from build123d import *

# Parameters (mm, degrees)
F0_W     = 32
F0_H     = 50
F0_W_2   = 2
F0_H_2   = 6
F1_DEPTH = 10
F2_R     = 0.5


with BuildPart() as f1:
    # F0 (on Top) → F1 (new body)
    with BuildSketch(Plane.XY):
        Polygon((-17.5, 26.5), (-17.5, 25), (-17.5, -26.5), (17.5, -26.5), (17.5, 26.5), (-16, 26.5), align=None)
        Rectangle(F0_W, F0_H, mode=Mode.SUBTRACT)
        Polygon((-38, 25), (-17.5, 25), (-17.5, 26.5), (-39.5, 26.5), (-39.5, -8.5), (-38, -8.5), (-38, -2.5), align=None)
        with Locations((-37, -5.5)):
            Rectangle(F0_W_2, F0_H_2)
    extrude(amount=F1_DEPTH)

    # F2
    f2_edges = [f1.edges().sort_by_distance(p)[0] for p in [
        (-36, -2.5, 5),
        (-36, -8.5, 5),
        (17.5, -26.5, 5),
        (17.5, 26.5, 5),
        (-17.5, -26.5, 5),
        (-39.5, 26.5, 5),
        (-39.5, -8.5, 5),
    ]]
    fillet(f2_edges, radius=F2_R)


solid = f1.part
Work out the finished part from the listing and answer in its coordinate system (mm). A direction names the side the tool comes from. Round coordinates to 2 decimals unless told otherwise and drop trailing zeros. Write each loop counter-clockwise with the first axis right and the second up, starting at its lowest first coordinate (ties: lowest second). Pieces come first, ordered by that corner, then holes. Notation, with made-up numbers: (11, -15) -> (41, -15) arc R23 cw to (41, 17) -> close; hole circle Ø11 at (43.5, 52.25). An arc over 180 degrees is marked (long way). Answer as CSV lines item,"result". Start each with the question number.
(1) The part is cut by section A-A, the plane y = -13.5. Give the vertices of the cut face in (x, z).
(2) This flat-tipped pin is pushed along its axis until it touches: pin 1 (3 mm diameter, centred on x = -37, z = 6.5, fed in from -Y). Where does it stop, or does it pass through?
(3) The part is cut by section D-D, the plane y = 13.5. Give the vertices of the cut face in (x, z).
(4) The part is cut by section B-B, the plane x = -2. Give the vertices of the cut face in (y, z).
(5) The part is cut by section C-C, the plane z = 8. Give the vertices of the cut face in (x, y), then the cut area to 3 significant figures.
(6) A tool of negligible diameter and unlimited length cuts with its end or side. For faces 4 (the flat face through (-17.5, 0, 5)), 5 (the flat face through (-17, 4, 10)), 6 (the flat face through (-37, -2.5, 5)), 7 (the flat face through (-38, -8.5, 5)), from which of +Z, -Z, +X, -X, +Y, -Y can it reach the whole face along a straight path? Write none if from no direction.
(7) The mould has two halves that part along X. Classify faces 1 (the flat face through (-39.5, 9, 5)), 2 (the flat face through (-17, 4, 0)), 3 (the flat face through (-16, 0, 5)): +X half, -X half, draft (parallel to the pull), parting line (faces both ways), or undercut.
(8) Find the intervals of material crossed by probe 1 along X at (y, z) = (15.5, 4.5); probe 2 along X at (y, z) = (-3, 3.75); probe 3 along Y at (x, z) = (3.5, 2.25), in increasing order.
Output values:
1,outline,"(-17.5, 0) -> (-16, 0) -> (-16, 10) -> (-17.5, 10) -> close; (16, 0) -> (17.5, 0) -> (17.5, 10) -> (16, 10) -> close"
2,pin 1,"stops at y = -8.5"
3,outline,"(-39.5, 0) -> (-38, 0) -> (-38, 10) -> (-39.5, 10) -> close; (-17.5, 0) -> (-16, 0) -> (-16, 10) -> (-17.5, 10) -> close; (16, 0) -> (17.5, 0) -> (17.5, 10) -> (16, 10) -> close"
4,outline,"(-26.5, 0) -> (-25, 0) -> (-25, 10) -> (-26.5, 10) -> close; (25, 0) -> (26.5, 0) -> (26.5, 10) -> (25, 10) -> close"
5,outline,"(-39.5, -8) arc R0.5 ccw to (-39, -8.5) -> (-36.5, -8.5) arc R0.5 ccw to (-36, -8) -> (-36, -3) arc R0.5 ccw to (-36.5, -2.5) -> (-38, -2.5) -> (-38, 25) -> (-17.5, 25) -> (-17.5, -26) arc R0.5 ccw to (-17, -26.5) -> (17, -26.5) arc R0.5 ccw to (17.5, -26) -> (17.5, 26) arc R0.5 ccw to (17, 26.5) -> (-39, 26.5) arc R0.5 ccw to (-39.5, 26) -> close; hole (-16, -25) -> (16, -25) -> (16, 25) -> (-16, 25) -> close"
5,area,"350 mm²"
6,face 4,"+Z, -Z, -Y"
6,face 5,"+Z, +X, -X, +Y, -Y"
6,face 6,"+Z, -Z"
6,face 7,"+Z, -Z, -X, -Y"
7,face 1,"-X half"
7,face 2,"draft"
7,face 3,"undercut"
8,probe 1,"x = -39.5 to -38, -17.5 to -16, 16 to 17.5"
8,probe 2,"x = -39.5 to -36, -17.5 to -16, 16 to 17.5"
8,probe 3,"y = -26.5 to -25, 25 to 26.5"
